from build123d import *

# Parameters (mm, degrees)
SKETCH1_W                = 90
SKETCH1_H                = 90
BOSS_EXTRUDE1_DEPTH      = 90
BOSS_EXTRUDE2_DEPTH      = 5
BOSS_EXTRUDE2_DEPTH_BACK = 90
SKETCH2_R                = 18.495149705
BOSS_EXTRUDE3_DEPTH      = 5
BOSS_EXTRUDE3_DEPTH_BACK = 90
SKETCH3_R                = 18.495149705
BOSS_EXTRUDE4_DEPTH      = 5
BOSS_EXTRUDE4_DEPTH_BACK = 90
SKETCH4_R                = 18.495149705
BOSS_EXTRUDE5_DEPTH      = 95.671853643
BOSS_EXTRUDE5_DEPTH_BACK = 90
SKETCH5_R                = 18.495149705
BOSS_EXTRUDE6_DEPTH      = 5
BOSS_EXTRUDE6_DEPTH_BACK = 90
SKETCH6_R                = 18.495149705
CUT_EXTRUDE1_DEPTH       = 90
SKETCH8_RX               = 9.776430477
SKETCH8_RY               = 3.640340221
CUT_EXTRUDE2_DEPTH       = 90
BOSS_EXTRUDE7_DEPTH      = 90
SKETCH10_R               = 29.435529535
SKETCH10_R_2             = 31.00879633
BOSS_EXTRUDE10_DEPTH     = 14
SKETCH11_W               = 90
SKETCH11_H               = 90
BOSS_EXTRUDE11_DEPTH     = 90
SKETCH14_W               = 90
SKETCH14_H               = 90
BOSS_EXTRUDE12_DEPTH     = 90
SKETCH15_W               = 90
SKETCH15_H               = 90
BOSS_EXTRUDE13_DEPTH     = 90


with BuildPart() as part:
    # Sketch1 → Boss-Extrude1 (new body)
    with BuildSketch(Plane.XY):
        Rectangle(SKETCH1_W, SKETCH1_H)
    extrude(amount=BOSS_EXTRUDE1_DEPTH)

    # Sketch2 → Boss-Extrude2 (add, two sides: drawn at the far end of the back side and taken through both)
    with BuildSketch(Plane(origin=(45, 0, 0), x_dir=(0, 0, -1), z_dir=(1, 0, 0)).offset(-BOSS_EXTRUDE2_DEPTH_BACK)):
        with Locations(Location((-42.533520746, 3.735944486, 0), (0, 0, 270))):
            Circle(SKETCH2_R)
    extrude(amount=BOSS_EXTRUDE2_DEPTH + BOSS_EXTRUDE2_DEPTH_BACK)

    # Sketch3 → Boss-Extrude3 (add, two sides: drawn at the far end of the back side and taken through both)
    with BuildSketch(Plane.XY.offset(90).offset(-BOSS_EXTRUDE3_DEPTH_BACK)):
        with Locations((-3.126781539, 1.624320901)):
            Circle(SKETCH3_R)
    extrude(amount=BOSS_EXTRUDE3_DEPTH + BOSS_EXTRUDE3_DEPTH_BACK)

    # Sketch4 → Boss-Extrude4 (add, two sides: drawn at the far end of the back side and taken through both)
    with BuildSketch(Plane(origin=(0, 45, 0), x_dir=(0, 0, -1), z_dir=(0, 1, 0)).offset(-BOSS_EXTRUDE4_DEPTH_BACK)):
        with Locations((-44.963029761, -1.140691585)):
            Circle(SKETCH4_R)
    extrude(amount=BOSS_EXTRUDE4_DEPTH + BOSS_EXTRUDE4_DEPTH_BACK)

    # Sketch5 → Boss-Extrude5 (add, two sides: drawn at the far end of the back side and taken through both)
    with BuildSketch(Plane.ZY.offset(45).offset(-BOSS_EXTRUDE5_DEPTH_BACK)):
        with Locations(Location((44.323215706, -3.480744369, 0), (0, 0, 90))):
            Circle(SKETCH5_R)
    extrude(amount=BOSS_EXTRUDE5_DEPTH + BOSS_EXTRUDE5_DEPTH_BACK)

    # Sketch6 → Boss-Extrude6 (add, two sides: drawn at the far end of the back side and taken through both)
    with BuildSketch(Plane(origin=(0, -45, 0), x_dir=(0, 0, -1), z_dir=(0, -1, 0)).offset(-BOSS_EXTRUDE6_DEPTH_BACK)):
        with Locations(Location((-43.114009277, -1.073204684, 0), (0, 0, 180))):
            Circle(SKETCH6_R)
    extrude(amount=BOSS_EXTRUDE6_DEPTH + BOSS_EXTRUDE6_DEPTH_BACK)

    # Sketch7 → Cut-Extrude1 (cut)
    with BuildSketch(Plane(origin=(0, 0, 0), x_dir=(-1, 0, 0), z_dir=(0, 0, -1))):
        Polygon((-28.802165797, 29.805616158), (-25.949050166, 35.352304143), (-29.326065052, 40.596518751), (-35.556195569, 40.294045375), (-38.4093112, 34.747357391), (-35.032296314, 29.503142782), align=None)
    extrude(amount=-CUT_EXTRUDE1_DEPTH, mode=Mode.SUBTRACT)

    # Sketch8 → Cut-Extrude2 (cut)
    with BuildSketch(Plane.XY.offset(90)):
        with Locations(Location((34.417640855, -28.6823815), (0, 0, -90))):
            Ellipse(SKETCH8_RX, SKETCH8_RY)
    extrude(amount=-CUT_EXTRUDE2_DEPTH, mode=Mode.SUBTRACT)

    # Sketch9 → Boss-Extrude7 (add)
    with BuildSketch(Plane(origin=(50, 0, 0), x_dir=(0, 0, -1), z_dir=(1, 0, 0))):
        with BuildLine():
            Line((-44.073528041, 6.623037359), (-44.073528041, 0))
            ThreePointArc((-44.073528041, 0), (-44.987170795, -0.913642754), (-45.900813549, 0))
            Line((-45.900813549, 0), (-45.900813549, 6.623037359))
            ThreePointArc((-45.900813549, 6.623037359), (-44.987170795, 7.536680113), (-44.073528041, 6.623037359))
        make_face()
    extrude(amount=BOSS_EXTRUDE7_DEPTH)

    # Sketch10 → Boss-Extrude10 (add)
    with BuildSketch(Plane(origin=(140, 6.623037359, 44.073528041), x_dir=(1, 0, 0), z_dir=(0, 1, 0))):
        with Locations((-8.425763271, 8.188123623)):
            Circle(SKETCH10_R)
        with Locations((-0.853882083, -0.578401306)):
            Circle(SKETCH10_R_2)
    extrude(amount=-BOSS_EXTRUDE10_DEPTH)

    # Sketch11 → Boss-Extrude11 (add)
    with BuildSketch(Plane.ZY.offset(140.671853643)):
        with Locations((46.274660301, 3.007862201)):
            Rectangle(SKETCH11_W, SKETCH11_H)
    extrude(amount=BOSS_EXTRUDE11_DEPTH)

    # Sketch14 → Boss-Extrude12 (add)
    with BuildSketch(Plane.XY.offset(91.274660301)):
        with Locations((-209.537955893, -13.069417981)):
            Rectangle(SKETCH14_W, SKETCH14_H)
    extrude(amount=BOSS_EXTRUDE12_DEPTH)

    # Sketch15 → Boss-Extrude13 (add)
    with BuildSketch(Plane.ZY.offset(230.671853643)):
        with Locations((56.117901354, 35.887776579)):
            Rectangle(SKETCH15_W, SKETCH15_H)
    extrude(amount=BOSS_EXTRUDE13_DEPTH)


solid = part.part
Read the model definition and answer for the solid it produces. Units are mm, in the model's axes. A direction names the side the tool comes from. Coordinates: 2 decimals unless noted, no trailing zeros. Write each loop counter-clockwise with the first axis right and the second up, starting at its lowest first coordinate (ties: lowest second). Pieces come first, ordered by that corner, then holes. Notation, with made-up numbers: M 7.25,63 L 30.25,63 A33 cw 30.25,92 Z; hole C -34,-37 d1. An arc over 180 degrees is marked long. Use a Markdown table: item, result.
Q1. Straight lines are drawn through the part: L1, parallel to X at y = 20.5, z = 29.5; L2, parallel to Y at x = -227, z = 72; L3, parallel to Z at x = -167, y = -43.5. For each, find the intervals that lie inside material, in ascending order. Write a range as [from, to].
Answer block:
| item | result |
|---|---|
| L1 | x = [-320.67, -140.67], [-45, 45] |
| L2 | y = [-41.99, 48.01] |
| L3 | z = [91.27, 181.27] |
Q2. The part is cut by section A-A, the plane x = -203. Write down the section's boundary in (y, z).
Answer block:
| item | result |
|---|---|
| outline | M -58.07,91.27 L -41.99,91.27 L -41.99,1.27 L 48.01,1.27 L 48.01,91.27 L 31.93,91.27 L 31.93,181.27 L -58.07,181.27 Z |
Q3. The part is cut by section D-D, the plane z = 85. Give the number of separate pieces and of enclosed holes in the cut face, then the cut area to 3 significant figures.
Answer block:
| item | result |
|---|---|
| separate pieces | 2 |
| enclosed holes | 2 |
| area | 24,100 mm2 |
Q4. The part is cut by section B-B, the plane y = 55.5. Write down the section's boundary in (x, z), then the cut area to 3 significant figures.
Answer block:
| item | result |
|---|---|
| outline | M -320.67,11.12 L -230.67,11.12 L -230.67,101.12 L -320.67,101.12 Z |
| area | 8,100 mm2 |
Q5. The part is cut by section C-C, the plane z = 131.5. Write down the section's boundary in (x, y).
Answer block:
| item | result |
|---|---|
| outline | M -254.54,-58.07 L -164.54,-58.07 L -164.54,31.93 L -254.54,31.93 Z |
Q6. Each of these flat-tipped pins is pushed along its axis until it touches: pin 1 Ø18.5 at (x, z) = (0, 50) entering from +Y; pin 2 Ø1.5 at (x, z) = (-234.5, 84) entering from -Y; pin 3 Ø18.5 at (x, y) = (-5.5, -6.5) entering from +Z. Where does it stop, or does it pass through?
Answer block:
| item | result |
|---|---|
| pin 1 | stops at y = 50 |
| pin 2 | stops at y = -9.11 |
| pin 3 | stops at z = 95 |
Q7. Which of the six approach directions +Z, -Z, +X, -X, +Y, -Y give full straight-line access (tool end or side, diameter ignored) to faces 4 (the face through (136, 6.623, 41)), 5 (the face through (-1.886, -47.465, 24.637)), 6 (the face through (-185, -41.992, 46)), 7 (the face through (-185, 2, 1.275)), 8 (the face through (-17.804, -9.63, 92.465))?
Answer block:
| item | result |
|---|---|
| face 4 | +X, +Y |
| face 5 | -Y |
| face 6 | -Z, -X, -Y |
| face 7 | -Z, -X, +Y, -Y |
| face 8 | +Z |
Q8. Determine the mould class of faces 1 (the face through (-21, 45, 44)), 2 (the face through (-210, -12, 181.275)), 3 (the face through (-320.672, 37, 55)) for opening direction X: released by +X, released by -X, zero draft, split by the parting line, or undercut.
Answer block:
| item | result |
|---|---|
| face 1 | undercut |
| face 2 | zero draft |
| face 3 | released by -X |
